```python
from build123d import *

# Parameters (mm, degrees)
SKICA1_W                 = 54.6
SKICA1_H                 = 54.6
P_IDAT_VYSUNUT_M2_DEPTH  = 3
SKICA5_W                 = 5
SKICA5_H                 = 24.8
ODEBRAT_VYSUNUT_M3_DEPTH = 1
SKICA14_W                = 52.6
SKICA14_H                = 1
P_IDAT_VYSUNUT_M9_DEPTH  = 15
SKICA17_R                = 2
ODEBRAT_VYSUNUT_M8_DEPTH = 7
SKICA19_W                = 7.8
SKICA19_H                = 7.8
P_IDAT_VYSUNUT_M10_DEPTH = 18
SKICA20_R                = 2.4
ODEBRAT_VYSUNUT_M9_DEPTH = 1.7
ZAOBLIT1_R               = 3
ZAOBLIT2_R               = 15
ZAOBLIT3_R               = 20


with BuildPart() as part:
    # Skica1 → Přidat vysunutím2 (new body)
    with BuildSketch(Plane.XY):
        Rectangle(SKICA1_W, SKICA1_H)
    extrude(amount=P_IDAT_VYSUNUT_M2_DEPTH)

    # Skica5 → Odebrat vysunutím3 (cut)
    with BuildSketch(Plane(origin=(0, 0, 0), x_dir=(-1, 0, 0), z_dir=(0, 0, -1))):
        with Locations((0, 14.9)):
            Rectangle(SKICA5_W, SKICA5_H)
        Polygon((27.3, 2.5), (2.5, 2.5), (-2.5, 2.5), (-2.5, -2.5), (27.3, -2.5), align=None)
    extrude(amount=-ODEBRAT_VYSUNUT_M3_DEPTH, mode=Mode.SUBTRACT)

    # Skica14 → Přidat vysunutím9 (add)
    with BuildSketch(Plane.XY.offset(3)):
        Polygon((27.3, 27.3), (-27.3, 27.3), (-27.3, -27.3), (-26.3, -27.3), (-26.3, -26.3), (-26.3, 26.3), (26.3, 26.3), (26.3, -26.3), (26.3, -27.3), (27.3, -27.3), align=None)
        with Locations((0, -26.8)):
            Rectangle(SKICA14_W, SKICA14_H)
    extrude(amount=P_IDAT_VYSUNUT_M9_DEPTH)

    # Skica17 → Odebrat vysunutím8 (cut)
    with BuildSketch(Plane(origin=(0, 0, 1), x_dir=(-1, 0, 0), z_dir=(0, 0, -1))):
        with Locations((20.3, 0)):
            Circle(SKICA17_R)
        with Locations((0, 20.3)):
            Circle(SKICA17_R)
    extrude(amount=-ODEBRAT_VYSUNUT_M8_DEPTH, mode=Mode.SUBTRACT)

    # Skica19 → Přidat vysunutím10 (add)
    with BuildSketch(Plane(origin=(0, 0, 0), x_dir=(-1, 0, 0), z_dir=(0, 0, -1))):
        with Locations((-23.4, 23.4)):
            Rectangle(SKICA19_W, SKICA19_H)
        with Locations((23.4, 23.4)):
            Rectangle(SKICA19_W, SKICA19_H)
        with Locations((-23.4, -23.4)):
            Rectangle(SKICA19_W, SKICA19_H)
        with Locations((23.4, -23.4)):
            Rectangle(SKICA19_W, SKICA19_H)
    extrude(amount=-P_IDAT_VYSUNUT_M10_DEPTH)

    # Skica20 → Odebrat vysunutím9 (cut)
    with BuildSketch(Plane.XY.offset(18)):
        with Locations((-23.4, -23.4)):
            Circle(SKICA20_R)
        with Locations((-23.4, 23.4)):
            Circle(SKICA20_R)
        with Locations((23.400280565, 23.4)):
            Circle(SKICA20_R)
        with Locations((23.400280565, -23.4)):
            Circle(SKICA20_R)
    extrude(amount=-ODEBRAT_VYSUNUT_M9_DEPTH, mode=Mode.SUBTRACT)

    # Zaoblit1
    zaoblit1_edges = [part.edges().sort_by_distance(p)[0] for p in [
        (-19.5, 19.5, 10.5),
        (19.5, -19.5, 10.5),
        (-19.5, -19.5, 10.5),
        (19.5, 19.5, 10.5),
    ]]
    fillet(zaoblit1_edges, radius=ZAOBLIT1_R)

    # Zaoblit2
    zaoblit2_edges = [part.edges().sort_by_distance(p)[0] for p in [
        (-2.5, 2.5, 0.5),
    ]]
    fillet(zaoblit2_edges, radius=ZAOBLIT2_R)

    # Zaoblit3
    zaoblit3_edges = [part.edges().sort_by_distance(p)[0] for p in [
        (2.5, -2.5, 0.5),
    ]]
    fillet(zaoblit3_edges, radius=ZAOBLIT3_R)


solid = part.part
```
Can you work these out from the model? Positions are in its coordinate system, mm. A direction names the side the tool comes from. Coordinates: 2 decimals unless noted, no trailing zeros. Loops run counter-clockwise (first coordinate to the right, second up) from the corner with the lowest first, then second, coordinate; pieces in that order, holes last. Notation, with made-up numbers: (4, 39) - (23, 39) arc R14 cw to (23, 66) - close; hole circle Ø5 at (21.25, -29.5). An arc over 180 degrees is marked (long way). Answer as CSV lines item,"result". Start each with the question number.
1) I need wall thicknesses on line 1 (Y direction, x = 10.5, z = 10.5); line 2 (Y direction, x = -23.4, z = 17.55). Which ranges of each line are inside material? Lowest first, please. Write a range as from..to.
2) Thinking about a two-plate mould opening in Y: for faces 4 (the cylindrical face through (-1.075, 21.986, 1.986)), 5 (the flat face through (-15, 15, 0)), 6 (the flat face through (0, -27.3, 9)), 7 (the flat face through (0, 27.3, 9)), which applies, pulls with the +Y half, pulls with the -Y half, needs draft (parallel to the pull), parting line crosses it, or undercut?
3) Suppose I cut it at D-D (y = -23.4). Please give me the cut outline in (x, z), plus the area to 3 significant figures.
4) Which directions (+Z, -Z, +X, -X, +Y, -Y) give clear straight access to the entire face, cutting with the end or side of a thin tool? Please do faces 1 (the flat face through (0, 26.3, 10)), 2 (the flat face through (-5, 8, 1)), 3 (the flat face through (-27.3, 0, 9)).
5) Suppose I cut it at A-A (z = 11.75). Please give me the cut outline in (x, y), plus the area to 3 significant figures.
6) Suppose I cut it at C-C (x = 0). Please give me the cut outline in (y, z), plus the area to 3 significant figures.
7) For pin 1 (2 mm diameter, centred on x = -14.5, y = 12.5, fed in from +Z); pin 2 (1.4 mm diameter, centred on x = 22.5, y = 22.5, fed in from +Z); pin 3 (2.5 mm diameter, centred on x = -20.3, y = 0, fed in from +Z), each with a flat end and sliding along its axis, tell me the tip position at first contact or that it passes through.
8) Suppose I cut it at B-B (y = 0). Please give me the cut outline in (x, z), plus the area to 3 significant figures.
Check result:
1,line 1,"y = -27.3..-26.3, 26.3..27.3"
1,line 2,"y = -27.3..-25.8, -21..-19.5, 19.5..21, 25.8..27.3"
2,face 4,"undercut"
2,face 5,"needs draft"
2,face 6,"pulls with the -Y half"
2,face 7,"pulls with the +Y half"
3,outline,"(-27.3, 0) - (27.3, 0) - (27.3, 18) - (25.8, 18) - (25.8, 16.3) - (21, 16.3) - (21, 18) - (19.5, 18) - (19.5, 3) - (-19.5, 3) - (-19.5, 18) - (-21, 18) - (-21, 16.3) - (-25.8, 16.3) - (-25.8, 18) - (-27.3, 18) - close"
3,area,"381 mm²"
4,face 1,"+Z"
4,face 2,"-Z"
4,face 3,"+Z, -Z, -X, +Y, -Y"
5,outline,"(-27.3, -27.3) - (27.3, -27.3) - (27.3, 27.3) - (-27.3, 27.3) - close; hole (-26.3, -19.5) - (-22.5, -19.5) arc R3 cw to (-19.5, -22.5) - (-19.5, -26.3) - (19.5, -26.3) - (19.5, -22.5) arc R3 cw to (22.5, -19.5) - (26.3, -19.5) - (26.3, 19.5) - (22.5, 19.5) arc R3 cw to (19.5, 22.5) - (19.5, 26.3) - (-19.5, 26.3) - (-19.5, 22.5) arc R3 cw to (-22.5, 19.5) - (-26.3, 19.5) - close"
5,area,"392 mm²"
6,outline,"(-27.3, 0) - (7.82, 0) - (7.82, 1) - (18.3, 1) - (18.3, 3) - (-26.3, 3) - (-26.3, 18) - (-27.3, 18) - close; (22.3, 1) - (27.3, 1) - (27.3, 18) - (26.3, 18) - (26.3, 3) - (22.3, 3) - close"
6,area,"166 mm²"
7,pin 1,"stops at z = 3"
7,pin 2,"stops at z = 16.3"
7,pin 3,"passes through"
8,outline,"(-27.3, 1) - (-22.3, 1) - (-22.3, 3) - (-26.3, 3) - (-26.3, 18) - (-27.3, 18) - close; (-18.3, 1) - (-7.82, 1) - (-7.82, 0) - (27.3, 0) - (27.3, 18) - (26.3, 18) - (26.3, 3) - (-18.3, 3) - close"
8,area,"166 mm²"
